Geometry check sheet. Reference: drawing and pictorial views, mm from the part's lowest x, y, z. Round coordinates to 2 decimals unless told otherwise and drop trailing zeros. Write each loop counter-clockwise with the first axis right and the second up, starting at its lowest first coordinate (ties: lowest second). Pieces come first, ordered by that corner, then holes. Notation, with made-up numbers: (-36.5, 85) -> (-2.5, 85) arc R21 ccw to (-2.5, 94) -> close; hole circle Ø10 at (19, -10). An arc over 180 degrees is marked (long way). Write item = value, one per line.
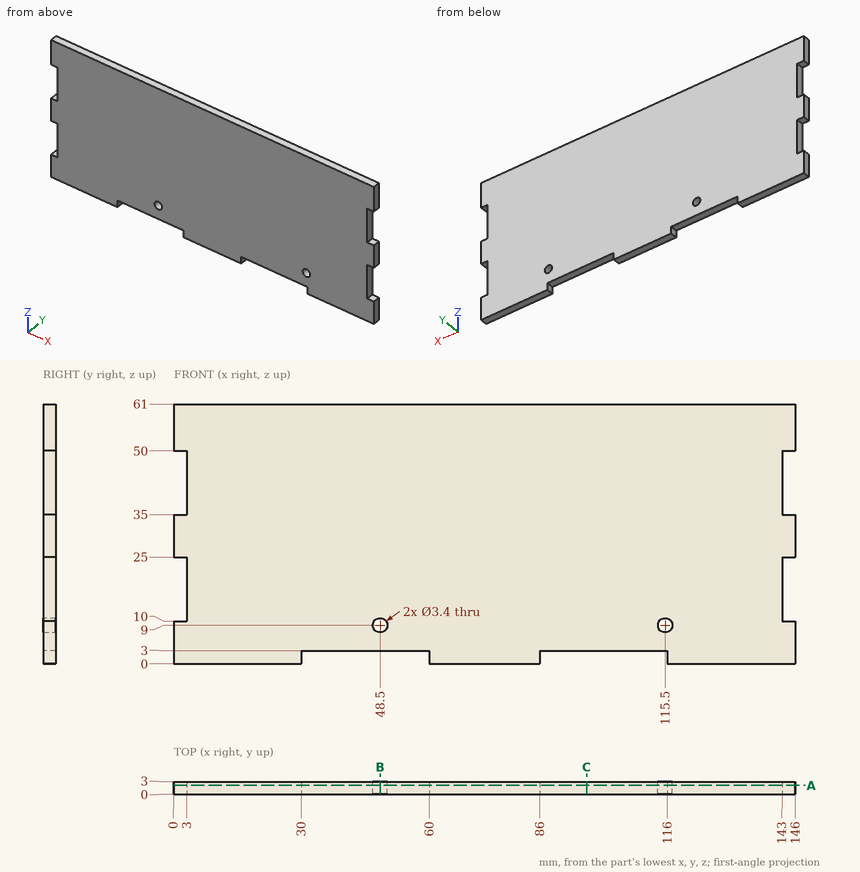
(1) Sectioned sample at C-C on x = 97. Enter the section's corners in (y, z).
Worked answers:
outline = (0, 3) -> (3, 3) -> (3, 61) -> (0, 61) -> close
(2) Go/stop test with flat-tipped pins: P1, Ø3, axis at x = 48.5, z = 9, coming from the -Y side; P2, Ø1.5, axis at y = 0.5, z = 15.5, coming from the -X side; P3, Ø0.9, axis at x = 42, y = 1, coming from the -Z side; P4, Ø0.9, axis at y = 2, z = 39.5, coming from the +X side. Record where each tip stops, or that it passes through.
Worked answers:
P1 = through
P2 = 3
P3 = 3
P4 = 143
(3) Sectioned sample at B-B on x = 48.5. Enter the section's corners in (y, z), then the cut area to 3 significant figures.
Worked answers:
outline = (0, 3) -> (3, 3) -> (3, 7.3) -> (0, 7.3) -> close; (0, 10.7) -> (3, 10.7) -> (3, 61) -> (0, 61) -> close
area = 164 mm²
(4) Sectioned sample at A-A on y = 2.1. Count the separate pieces of the cut face and the enclosed holes in it, then the cut area to 3 significant figures.
Worked answers:
separate_pieces = 1
enclosed_holes = 2
area = 8,530 mm²
(5) Material ranges on L1, parallel to X at y = 0.85, z = 9; L2, parallel to Z at x = 48.5, y = 0.8; L3, parallel to X at y = 0.4, z = 36, recorded low to high. Write a range as [from, to].
Worked answers:
L1 = [0, 46.8], [50.2, 113.8], [117.2, 146]
L2 = [3, 7.3], [10.7, 61]
L3 = [3, 143]
